Part model, mm, in its own coordinate system. Face numbers are marked on the shaded views. A direction names the side the tool comes from. Round coordinates to 2 decimals unless told otherwise and drop trailing zeros. Order: outer loops, then holes, each group sorted by start corner. A loop starts at its lowest first (then second) coordinate and runs counter-clockwise, first axis right, second up. Notation, with made-up numbers: (24, 24.25) -> (55, 24.25) arc R7 cw to (55, 35.25) -> close; hole circle Ø7 at (46.5, 31.25). An arc over 180 degrees is marked (long way). Use CSV: the item, a comma, the result in double quotes.
```python
from build123d import *

# Parameters (mm, degrees)
F0_W     = 31.75
F0_H     = 12.7
F1_DEPTH = 25.4
F3_DEPTH = 25.4
F5_DEPTH = 25.4
F7_DEPTH = 25.4
F8_R     = 12.69999


# Not quite as in the source:
# - a fillet or chamfer is up to 0.001 mm smaller than in the source, because OpenCascade refuses the exact size


with BuildPart() as f1:
    # F0 (on Top) → F1 (new body)
    with BuildSketch(Plane.XY):
        Polygon((0, 12.7), (0, 0), (25.4, 0), (25.4, 12.7), (25.4, 44.45), (0, 44.45), align=None)
        with Locations((-15.875, 6.35)):
            Rectangle(F0_W, F0_H)
        with Locations((41.275, 6.35)):
            Rectangle(F0_W, F0_H)
    extrude(amount=F1_DEPTH)

    # F2 (on face) → F3 (cut)
    with BuildSketch(Plane.YZ.offset(25.4)):
        with BuildLine():
            ThreePointArc((38.1, 12.7), (36.2401280605, 17.1901280605), (31.75, 19.05))
            ThreePointArc((31.75, 19.05), (27.2598719395, 8.2098719395), (38.1, 12.7))
        make_face()
    extrude(amount=-F3_DEPTH, mode=Mode.SUBTRACT)

    # F4 (on face) → F5 (cut)
    with BuildSketch(Plane(origin=(0, 12.7, 0), x_dir=(-1, 0, 0), z_dir=(0, 1, 0))):
        with BuildLine():
            ThreePointArc((-44.45, 19.05), (-48.9401280605, 8.2098719395), (-38.1, 12.7))
            ThreePointArc((-38.1, 12.7), (-39.9598719395, 17.1901280605), (-44.45, 19.05))
        make_face()
    extrude(amount=-F5_DEPTH, mode=Mode.SUBTRACT)

    # F6 (on face) → F7 (cut)
    with BuildSketch(Plane(origin=(0, 12.7, 0), x_dir=(-1, 0, 0), z_dir=(0, 1, 0))):
        with BuildLine():
            ThreePointArc((19.05, 6.35), (23.5401280605, 8.2098719395), (25.4, 12.7))
            ThreePointArc((25.4, 12.7), (14.5598719395, 17.1901280605), (19.05, 6.35))
        make_face()
    extrude(amount=-F7_DEPTH, mode=Mode.SUBTRACT)

    # F8 (radius 12.7 in the source; OpenCascade refuses exactly that, so slightly less here)
    f8_edges = [f1.edges().sort_by_distance(p)[0] for p in [
        (57.15, 6.35, 25.4),
        (57.15, 6.35, 0),
        (12.7, 44.45, 25.4),
        (12.7, 44.45, 0),
        (-31.75, 6.35, 0),
        (-31.75, 6.35, 25.4),
    ]]
    fillet(f8_edges, radius=F8_R)


solid = f1.part
```
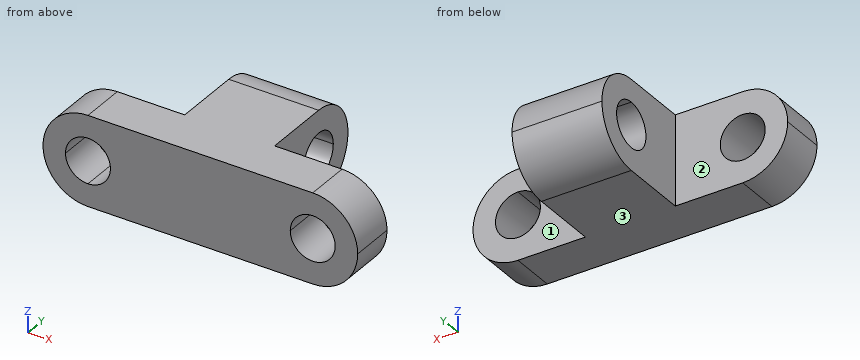
(1) Which spindle directions (+Z, -Z, +X, -X, +Y, -Y) get a long thin tool onto all of the face, cutting with end or side? Do the marked faces 1, 2 and 3. Say none if no direction does.
Reply:
face 1,"+Z, -Z, +X, +Y"
face 2,"+Z, -Z, -X, +Y"
face 3,"-Z, +X, -X, +Y, -Y"
(2) Probe probe 1 along X at (y, z) = (7, 13); probe 2 along X at (y, z) = (4, 12.7); probe 3 along Z at (x, y) = (44, 7). List the from-to ranges inside material, lowest first. Write a range as [from, to].
Reply:
probe 1,"[-31.75, -25.39], [-12.71, 38.11], [50.79, 57.15]"
probe 2,"[-31.75, -25.4], [-12.7, 38.1], [50.8, 57.15]"
probe 3,"[0, 6.37], [19.03, 25.4]"
(3) Cut at B-B, the plane y = 11.5. State how many separate pieces and enclosed holes the cut face has, then the cut area to 3 significant figures.
Reply:
separate pieces,"1"
enclosed holes,"2"
area,"1,870 mm2"
(4) Drop flat-ended pins along their axis: P1, Ø14.5, axis at x = -19.05, z = 12.7, coming from the +Y side; P2, Ø2, axis at y = 39.5, z = 9, coming from the -X side; P3, Ø2, axis at y = 12.5, z = 6, coming from the +X side. Give the stop position or say it passes through.
Reply:
P1,"y = 12.7"
P2,"x = 0"
P3,"x = 55.8"
(5) Cut at D-D, the plane x = -23. Give the cut face in (y, z).
Reply:
outline,"(0, 0.63) -> (12.7, 0.63) -> (12.7, 7.73) -> (0, 7.73) -> close; (0, 17.67) -> (12.7, 17.67) -> (12.7, 24.77) -> (0, 24.77) -> close"
(6) Cut at C-C, the plane z = 8. Give the cut face in (x, y), then the cut area to 3 significant figures.
Reply:
outline,"(-30.85, 0) -> (-23.32, 0) -> (-23.32, 12.7) -> (-30.85, 12.7) -> close; (-14.78, 0) -> (40.18, 0) -> (40.18, 12.7) -> (25.4, 12.7) -> (25.4, 27.48) -> (0, 27.48) -> (0, 12.7) -> (-14.78, 12.7) -> close; (0, 36.02) -> (25.4, 36.02) -> (25.4, 43.55) -> (0, 43.55) -> close; (48.72, 0) -> (56.25, 0) -> (56.25, 12.7) -> (48.72, 12.7) -> close"
area,"1,460 mm2"
